Verification items for the finished model (mm, model axes). Face numbers are marked on the shaded views. A direction names the side the tool comes from. Give positions to 0.01 mm unless a question says otherwise; leave off trailing zeros. Write each loop counter-clockwise with the first axis right and the second up, starting at its lowest first coordinate (ties: lowest second). Pieces come first, ordered by that corner, then holes. Notation, with made-up numbers: (-30, 41) - (14, 41) arc R7 ccw to (14, 51) - close; hole circle Ø8 at (31.5, -29.75). An arc over 180 degrees is marked (long way). Answer as a JSON object with one key per item and string values. Group by question number.
Item 1: Sectioned sample at A-A, the plane z = 8.5. Record the boundary of the cut face in (x, y).
Item 2: Draft check along Z on the marked faces 3, 4, 5 and 6. Enter one of: +Z half, -Z half, draft (parallel to the pull), parting line (faces both ways), or undercut.
Item 3: Scan lines: line 1 along X through (y, z) = (54, 35); line 2 along Y through (x, z) = (138, 56.5); line 3 along Y through (x, z) = (92.5, 77.5). Record each from-to range of solid material in increasing order. Write a range as [from, to].
Item 4: Sectioned sample at B-B, the plane y = 18. Record the boundary of the cut face in (x, z), and give its area (3 significant figures).
Item 5: Go/stop test with flat-tipped pins: pin 1 (6 mm diameter, centred on x = 60, z = 34, fed in from -Y); pin 2 (2 mm diameter, centred on y = 34, z = 76.5, fed in from +X). Record where each tip stops, or that it passes through.
Item 6: Tool access check on the marked faces 1 and 2. Record the directions out of +Z, -Z, +X, -X, +Y, -Y that give a thin tool (end or side, any length) a straight path to the whole face; none if there is none.
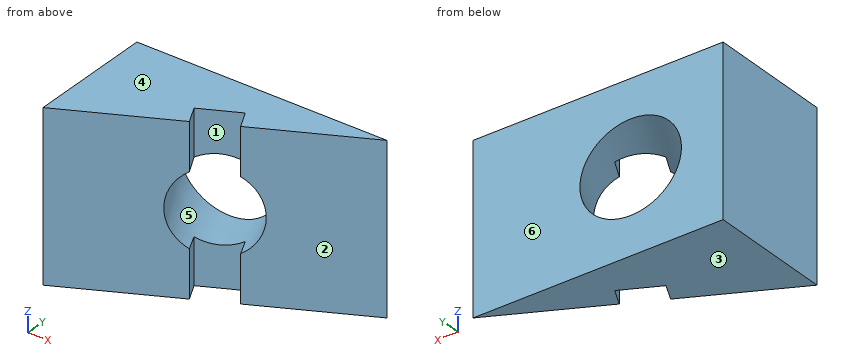
```python
from build123d import *

# Parameters (mm, degrees)
F1_DEPTH = 101.6
F2_W     = 25.4
F2_H     = 101.6
F3_DEPTH = 12.7
F5_DEPTH = 141.478
F5_TAPER = -3


with BuildPart() as f1:
    # F0 (on Top) → F1 (new body)
    with BuildSketch(Plane.XY):
        Polygon((0, 76.2), (0, 0), (152.4, 76.2), align=None)
    extrude(amount=F1_DEPTH)

    # F2 (on face) → F3 (cut)
    with BuildSketch(Plane(origin=(0, 0, 0), x_dir=(0.894427191, 0.4472135955, 0), z_dir=(0.4472135955, -0.894427191, 0))):
        with Locations((85.1941899427, 50.8)):
            Rectangle(F2_W, F2_H)
    extrude(amount=-F3_DEPTH, mode=Mode.SUBTRACT)

    # F4 (on face) → F5 (cut)
    with BuildSketch(Plane(origin=(0, 0, 0), x_dir=(0.894427191, 0.4472135955, 0), z_dir=(0.4472135955, -0.894427191, 0))):
        with BuildLine():
            ThreePointArc((72.4941899427, 28.8029547439), (97.8941899427, 28.8029547439), (110.5941899427, 50.8))
            ThreePointArc((110.5941899427, 50.8), (97.8941899427, 72.7970452561), (72.4941899427, 72.7970452561))
            Line((72.4941899427, 72.7970452561), (72.4941899427, 28.8029547439))
        make_face()
        with BuildLine():
            Line((72.4941899427, 28.8029547439), (72.4941899427, 72.7970452561))
            ThreePointArc((72.4941899427, 72.7970452561), (59.7941899427, 50.8), (72.4941899427, 28.8029547439))
        make_face()
    extrude(amount=-F5_DEPTH, taper=F5_TAPER, mode=Mode.SUBTRACT)


solid = f1.part
```
Geometry check:
{
 "1": {"outline": "(0, 0) - (64.84, 32.42) - (59.16, 43.78) - (81.88, 55.14) - (87.56, 43.78) - (152.4, 76.2) - (0, 76.2) - close"},
 "2": {"face 3": "-Z half", "face 4": "+Z half", "face 5": "undercut", "face 6": "draft"},
 "3": {"line 1": "[0, 43.91], [91.05, 108]", "line 2": "[69, 76.2]", "line 3": "[46.25, 76.2]"},
 "4": {"outline": "(0, 0) - (36, 0) - (36, 101.6) - (0, 101.6) - close", "area": "3,660 mm^2"},
 "5": {"pin 1": "y = 28.5", "pin 2": "x = 64.55"},
 "6": {"face 1": "+Z, -Z", "face 2": "+Z, -Z, +X, -Y"}
}
